from build123d import *

# Parameters (mm, degrees)
ESQUISSE1_W                  = 80
ESQUISSE1_H                  = 20
BOSS_EXTRU_1_DEPTH           = 5
CONG_1_R                     = 4
ENL_V_MAT_EXTRU_1_DEPTH      = 83.613558209
ENL_V_START                  = -5
ENL_V_MAT_EXTRU_2_DEPTH      = 5
ESQUISSE11_W                 = 13.611032385
ESQUISSE11_H                 = 17.64061434
BOSS_EXTRU_8_DEPTH           = 5
ENL_V_MAT_EXTRU_3_DEPTH      = 83.613558336
ENL_V_MAT_EXTRU_3_DEPTH_BACK = 83.613558336
ESQUISSE13_R                 = 3
ENL_V_MAT_EXTRU_4_DEPTH      = 33
BOSS_EXTRU_9_DEPTH           = 2.5


# Read off the part's stored shape, not the designer's step: Enlèv. mat.-Extru.2
with BuildPart() as part:
    # Esquisse1 → Boss.-Extru.1 (new body)
    with BuildSketch(Plane.XY):
        with Locations((40, -10)):
            Rectangle(ESQUISSE1_W, ESQUISSE1_H)
    extrude(amount=BOSS_EXTRU_1_DEPTH)

    # Congé1
    cong_1_edges = [part.edges().sort_by_distance(p)[0] for p in [
        (0, 0, 2.5),
        (80, 0, 2.5),
        (80, -20, 2.5),
        (0, -20, 2.5),
    ]]
    fillet(cong_1_edges, radius=CONG_1_R)

    # Esquisse2 → Enlèv. mat.-Extru.1 (cut, through all)
    with BuildSketch(Plane.XY.offset(5)):
        Polygon((28.410040172, -2.300084773), (30.410040172, -2.300084773), (24.995829866, -18.113699025), (22.995829866, -18.113699025), align=None)
        Polygon((9.298142424, -2.198086037), (16.298142424, -2.198086037), (10.914062948, -18.113699025), (3.914062948, -18.113699025), align=None)
        Polygon((18.309829725, -2.300084773), (22.309829725, -2.300084773), (16.902589817, -18.093340154), (12.902589817, -18.093340154), align=None)
        Polygon((23.808061727, -2.300084773), (26.808061727, -2.300084773), (21.404325417, -18.111661936), (18.404325417, -18.111661936), align=None)
        Polygon((31.786127586, -2.300084773), (33.786127586, -2.300084773), (28.371917279, -18.113699025), (26.371917279, -18.113699025), align=None)
    extrude(amount=-ENL_V_MAT_EXTRU_1_DEPTH, mode=Mode.SUBTRACT)

    # Enlèv. mat.-Extru.2 outline → Enlèv. mat.-Extru.2 (cut)
    # profile 1 of 3: a face of its own
    with BuildSketch(Plane.XY.offset(5).offset(ENL_V_START)):
        with BuildLine():
            add(Edge.make_bspline(
                [(75.686567024, -16.611023442), (75.678643784, -16.704663886), (75.663447013, -16.884266233), (75.563839443, -17.132408637), (75.415616385, -17.347383223), (75.204262037, -17.518269705), (74.945020643, -17.657920052), (74.629763147, -17.753299102), (74.263391467, -17.817731699), (74.000846179, -17.830167685), (73.861085096, -17.83678775)],
                knots=[0, 0, 0, 0, 0.114098337, 0.218840581, 0.322174175, 0.429434412, 0.547100708, 0.679564678, 0.829422238, 1, 1, 1, 1], degree=3))
            Line((75.686567024, -16.611023442), (75.686567024, -9.411486545))
            Line((75.686567024, -9.411486545), (69.882470639, -9.411486545))
            Line((69.882470639, -9.411486545), (69.882470639, -11.283775701))
            Line((69.882470639, -11.283775701), (72.316446542, -11.283775701))
            Line((72.316446542, -11.283775701), (72.316446542, -15.777269677))
            Line((72.316446542, -15.777269677), (67.822952566, -15.777269677))
            Line((67.822952566, -15.777269677), (67.822952566, -4.356305822))
            Line((67.822952566, -4.356305822), (72.316446542, -4.356305822))
            Line((72.316446542, -4.356305822), (72.316446542, -6.977510641))
            Line((72.316446542, -6.977510641), (75.686567024, -6.977510641))
            Line((75.686567024, -6.977510641), (75.686567024, -3.522552057))
            add(Edge.make_bspline(
                [(73.861085096, -2.29678775), (74.000846179, -2.303407815), (74.263391467, -2.3158438), (74.629763147, -2.380276397), (74.945020643, -2.475655447), (75.204262037, -2.615305794), (75.415616385, -2.786192276), (75.563839443, -3.001166862), (75.663447013, -3.249309266), (75.678643784, -3.428911613), (75.686567024, -3.522552057)],
                knots=[0, 0, 0, 0, 0.170577762, 0.320435322, 0.452899292, 0.570565588, 0.677825825, 0.781159419, 0.885901663, 1, 1, 1, 1], degree=3))
            Line((73.861085096, -2.29678775), (66.322195789, -2.29678775))
            add(Edge.make_bspline(
                [(64.452832084, -3.522552057), (64.460490101, -3.428813179), (64.475207603, -3.248661832), (64.578900626, -3.001012416), (64.72992953, -2.785012839), (64.947387079, -2.615412784), (65.212124175, -2.475706721), (65.534969931, -2.379572165), (65.910264022, -2.316247539), (66.179534857, -2.303527098), (66.322195789, -2.29678775)],
                knots=[0, 0, 0, 0, 0.112348161, 0.215915455, 0.318343111, 0.425762474, 0.543690884, 0.676356302, 0.828532073, 1, 1, 1, 1], degree=3))
            Line((64.452832084, -3.522552057), (64.452832084, -16.611023442))
            add(Edge.make_bspline(
                [(66.278314012, -17.83678775), (66.138552929, -17.830167685), (65.876007642, -17.817731699), (65.509635961, -17.753299102), (65.194378466, -17.657920052), (64.935137072, -17.518269705), (64.723782723, -17.347383223), (64.575559665, -17.132408637), (64.475952096, -16.884266233), (64.460755324, -16.704663886), (64.452832084, -16.611023442)],
                knots=[0, 0, 0, 0, 0.170577762, 0.320435322, 0.452899292, 0.570565588, 0.677825825, 0.781159419, 0.885901663, 1, 1, 1, 1], degree=3))
            Line((66.278314012, -17.83678775), (73.861085096, -17.83678775))
        make_face()
    # profile 2 of 3: a face of its own
    with BuildSketch(Plane.XY.offset(5).offset(ENL_V_START)):
        with BuildLine():
            add(Edge.make_bspline(
                [(59.247868229, -10.142849497), (59.250113416, -10.031576234), (59.255029992, -9.787906808), (59.301768342, -9.394005261), (59.364432817, -8.9400039), (59.423938248, -8.619443962), (59.455575307, -8.4490129)],
                knots=[0, 0, 0, 0, 0.195301478, 0.427676852, 0.695714808, 1, 1, 1, 1], degree=3))
            Line((59.247868229, -10.142849497), (59.247868229, -17.83678775))
            Line((59.247868229, -17.83678775), (62.617988711, -17.83678775))
            Line((62.617988711, -17.83678775), (62.617988711, -2.29678775))
            Line((62.617988711, -2.29678775), (59.481904374, -2.29678775))
            Line((59.481904374, -2.29678775), (55.68759338, -10.836181575))
            add(Edge.make_bspline(
                [(55.596904374, -11.538290009), (55.59815665, -11.492405908), (55.600881716, -11.392557927), (55.62162629, -11.229918497), (55.645376833, -11.040932864), (55.672949182, -10.907206292), (55.68759338, -10.836181575)],
                knots=[0, 0, 0, 0, 0.19413449, 0.422454333, 0.693254547, 1, 1, 1, 1], degree=3))
            add(Edge.make_bspline(
                [(55.506215368, -10.836181575), (55.516865461, -10.868148772), (55.54346006, -10.947974815), (55.561126156, -11.099283482), (55.582536457, -11.300899182), (55.59176432, -11.45336457), (55.596904374, -11.538290009)],
                knots=[0, 0, 0, 0, 0.142095852, 0.354830918, 0.640631437, 1, 1, 1, 1], degree=3))
            Line((55.506215368, -10.836181575), (51.711904374, -2.29678775))
            Line((51.711904374, -2.29678775), (48.575820036, -2.29678775))
            Line((48.575820036, -2.29678775), (48.575820036, -17.83678775))
            Line((48.575820036, -17.83678775), (51.945940518, -17.83678775))
            Line((51.945940518, -17.83678775), (51.945940518, -10.142849497))
            add(Edge.make_bspline(
                [(51.741158892, -8.4490129), (51.77262663, -8.62239324), (51.831532725, -8.946952903), (51.895555168, -9.402629403), (51.938009232, -9.793916754), (51.94345609, -10.033548389), (51.945940518, -10.142849497)],
                knots=[0, 0, 0, 0, 0.309420385, 0.579220093, 0.808073296, 1, 1, 1, 1], degree=3))
            Line((51.741158892, -8.4490129), (54.728045187, -16.338956424))
            Line((54.728045187, -16.338956424), (56.480390819, -16.338956424))
            Line((56.480390819, -16.338956424), (59.455575307, -8.4490129))
        make_face()
    # profile 3 of 3: a face of its own
    with BuildSketch(Plane.XY.offset(5).offset(ENL_V_START)):
        Polygon((44.119771843, -17.83678775), (47.489892325, -17.83678775), (43.019801964, -2.29678775), (39.439048952, -2.29678775), (34.945554976, -17.795831424), (34.945554976, -17.83678775), (38.315675458, -17.83678775), (39.023634795, -15.028354015), (43.41766341, -15.028354015), align=None)
        Polygon((41.217723651, -5.921422539), (42.923262054, -12.968835942), (39.488781633, -12.968835942), align=None, mode=Mode.SUBTRACT)
    extrude(amount=ENL_V_MAT_EXTRU_2_DEPTH, mode=Mode.SUBTRACT)

    # Esquisse11 → Boss.-Extru.8 (add)
    with BuildSketch(Plane.XY.offset(5)):
        with Locations((41.097921838, -10.121676789)):
            Rectangle(ESQUISSE11_W, ESQUISSE11_H)
    extrude(amount=-BOSS_EXTRU_8_DEPTH)

    # Esquisse12 → Enlèv. mat.-Extru.3 (cut, two sides: drawn at the far end of the back side and taken through both)
    with BuildSketch(Plane.XY.offset(5).offset(-ENL_V_MAT_EXTRU_3_DEPTH_BACK)):
        Polygon((35.786127586, -2.300084773), (42.786127586, -2.300084773), (48.111179633, -17.834694794), (46.111179633, -17.834694794), (44.102998893, -11.969278829), (35.786127586, -11.969278829), (37.115967439, -10.077108111), (43.455164056, -10.077108111), (41.446983316, -4.211692145), (37.138004335, -4.211692145), (32.518467193, -17.83678775), (30.518467193, -17.83678775), align=None)
    extrude(amount=ENL_V_MAT_EXTRU_3_DEPTH + ENL_V_MAT_EXTRU_3_DEPTH_BACK, mode=Mode.SUBTRACT)

    # Esquisse13 → Enlèv. mat.-Extru.4 (cut)
    with BuildSketch(Plane.XY.offset(5)):
        with Locations((4.24401363, -4.167068495)):
            Circle(ESQUISSE13_R)
    extrude(amount=-ENL_V_MAT_EXTRU_4_DEPTH, mode=Mode.SUBTRACT)

    # Esquisse14 → Boss.-Extru.9 (add)
    with BuildSketch(Plane(origin=(0, 0, 0), x_dir=(-1, 0, 0), z_dir=(0, 0, -1))):
        Polygon((-76.993137328, -1.775197305), (-76.993137328, -18.151298047), (-3.246627444, -18.151298047), (-8.832660873, -1.775197305), align=None)
    extrude(amount=-BOSS_EXTRU_9_DEPTH)


solid = part.part
The model under review builds one solid part; all positions refer to its coordinate system, in mm. A direction names the side the tool comes from. Give positions to 0.01 mm unless a question says otherwise; leave off trailing zeros. Loops run counter-clockwise (first coordinate to the right, second up) from the corner with the lowest first, then second, coordinate; pieces in that order, holes last. Notation, with made-up numbers: (58, 57.5) -> (104, 57.5) arc R18 cw to (104, 90.5) -> close; hole circle Ø10 at (2.5, 82). An arc over 180 degrees is marked (long way). Put each result on its own line as item: value. Start each with the question number.
1. For faces 1 (the face through (50, -17.837, 4)), 2 (the face through (39.4, -9.9, 5)), list the 3-axis set-ups (+Z, -Z, +X, -X, +Y, -Y) from which the entire face can be reached by the end or side of a thin tool; tool diameter is ignored.
2. We need section C-C on z = 4.25. State how many separate pieces and enclosed holes the cut face has, then the cut area to 3 significant figures.
3. Mouldability with a two-part tool opening along X and no side actions: class faces 3 (the face through (75.687, -13, 4)), 4 (the face through (1.141, -18.797, 2.535)), 5 (the face through (39, -10, 0)) as released by +X, released by -X, zero draft, split by the parting line, or undercut.
4. We need section D-D on x = 27.5. State the section outline as (y, z) points, then the cut area to 3 significant figures.
5. We need section B-B on x = 49.5. State the section outline as (y, z) points.
6. We need section A-A on x = 68.5. State the section outline as (y, z) points, then the cut area to 3 significant figures.
7. Wall thickness on probe 1 along Y at (x, z) = (62, 2.65); probe 2 along Y at (x, z) = (9.5, 4.85); probe 3 along Z at (x, y) = (19.5, -9.5): over which ranges is each line inside the solid? List them lowest first.
Determined:
1. face 1: +Z
1. face 2: +Z, +X, -X, +Y, -Y
2. separate pieces: 1
2. enclosed holes: 9
2. area: 919 mm^2
3. face 3: undercut
3. face 4: released by -X
3. face 5: zero draft
4. outline: (-20, 0) -> (0, 0) -> (0, 5) -> (-4.96, 5) -> (-4.96, 2.5) -> (-10.8, 2.5) -> (-10.8, 5) -> (-14.82, 5) -> (-14.82, 2.5) -> (-18.11, 2.5) -> (-18.11, 5) -> (-20, 5) -> close
4. area: 77.2 mm^2
5. outline: (-20, 0) -> (0, 0) -> (0, 5) -> (-2.3, 5) -> (-2.3, 2.5) -> (-17.84, 2.5) -> (-17.84, 5) -> (-20, 5) -> close
6. outline: (-20, 0) -> (0, 0) -> (0, 5) -> (-2.3, 5) -> (-2.3, 2.5) -> (-4.36, 2.5) -> (-4.36, 5) -> (-15.78, 5) -> (-15.78, 2.5) -> (-17.84, 2.5) -> (-17.84, 5) -> (-20, 5) -> close
6. area: 89.7 mm^2
7. probe 1: -20 to -17.84, -2.3 to 0
7. probe 2: -20 to -18.11, -2.2 to 0
7. probe 3: 0 to 2.5
